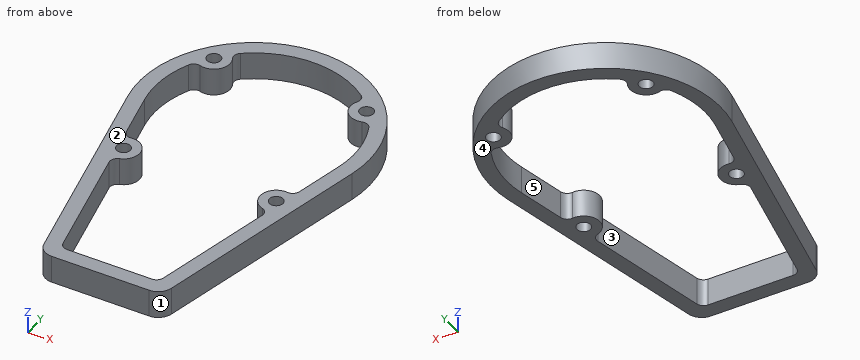
from build123d import *

# Parameters (mm, degrees)
SKETCH3_R           = 4.5
BOSS_EXTRUDE1_DEPTH = 18
FILLET1_R           = 5
FILLET2_R           = 5


with BuildPart() as part:
    # Sketch3 → Boss-Extrude1 (new body)
    with BuildSketch(Plane.XY):
        with BuildLine():
            Line((-31.929873349, -122.5), (31.929873349, -122.5))
            ThreePointArc((31.929873349, -122.5), (38.210043039, -120.281996444), (41.704324989, -114.611893732))
            Line((41.704324989, -114.611893732), (73.308387301, 31.660797012))
            ThreePointArc((73.308387301, 31.660797012), (0, 122.5), (-73.308387301, 31.660797012))
            Line((-73.308387301, 31.660797012), (-41.704324989, -114.611893732))
            ThreePointArc((-41.704324989, -114.611893732), (-38.210043039, -120.281996444), (-31.929873349, -122.5))
        make_face()
        with Locations((50, -12.5)):
            Circle(SKETCH3_R, mode=Mode.SUBTRACT)
        with Locations((50, 87.5)):
            Circle(SKETCH3_R, mode=Mode.SUBTRACT)
        with Locations((-50, 87.5)):
            Circle(SKETCH3_R, mode=Mode.SUBTRACT)
        with Locations((-50, -12.5)):
            Circle(SKETCH3_R, mode=Mode.SUBTRACT)
        with BuildLine():
            Line((-31.929873349, -112.5), (-51.284518999, -22.921132901))
            ThreePointArc((-51.284518999, -22.921132901), (-39.736825778, -10.282511582), (-55.472323677, -3.538768301))
            Line((-55.472323677, -3.538768301), (-63.533935661, 33.772690744))
            ThreePointArc((-63.533935661, 33.772690744), (-64.271528905, 57.204152316), (-56.648842383, 79.373322021))
            ThreePointArc((-56.648842383, 79.373322021), (-41.800877501, 80.940702001), (-43.531035666, 95.770580418))
            ThreePointArc((-43.531035666, 95.770580418), (0, 112.5), (43.531035666, 95.770580418))
            ThreePointArc((43.531035666, 95.770580418), (41.800877501, 80.940702001), (56.648842383, 79.373322021))
            ThreePointArc((56.648842383, 79.373322021), (64.271528905, 57.204152316), (63.533935661, 33.772690744))
            Line((63.533935661, 33.772690744), (55.472323677, -3.538768301))
            ThreePointArc((55.472323677, -3.538768301), (39.736825778, -10.282511582), (51.284518999, -22.921132901))
            Line((51.284518999, -22.921132901), (31.929873349, -112.5))
            Line((31.929873349, -112.5), (-31.929873349, -112.5))
        make_face(mode=Mode.SUBTRACT)
    extrude(amount=BOSS_EXTRUDE1_DEPTH)

    # Fillet1
    fillet1_edges = [part.edges().sort_by_distance(p)[0] for p in [
        (-31.929873349, -112.5, 9),
        (31.929873349, -112.5, 9),
    ]]
    fillet(fillet1_edges, radius=FILLET1_R)

    # Fillet2
    fillet2_edges = [part.edges().sort_by_distance(p)[0] for p in [
        (51.284518999, -22.921132901, 9),
        (55.472323677, -3.538768301, 9),
        (56.648842383, 79.373322021, 9),
        (43.531035666, 95.770580418, 9),
        (-43.531035666, 95.770580418, 9),
        (-56.648842383, 79.373322021, 9),
        (-55.472323677, -3.538768301, 9),
        (-51.284518999, -22.921132901, 9),
    ]]
    fillet(fillet2_edges, radius=FILLET2_R)


solid = part.part
Can you work these out from the model? Positions are in its coordinate system, mm. Face numbers are marked on the shaded views. A direction names the side the tool comes from. Give positions to 0.01 mm unless a question says otherwise; leave off trailing zeros. Loops run counter-clockwise (first coordinate to the right, second up) from the corner with the lowest first, then second, coordinate; pieces in that order, holes last. Notation, with made-up numbers: M 77.25,69.25 L 115.25,69.25 A25 cw 115.25,88.25 Z; hole C 30.5,32 d6. An arc over 180 degrees is marked long. One line per item, written item: value. Start each with the question number.
1) On a 3-axis mill with a long thin cutter (end or side, diameter ignored), from which of +Z, -Z, +X, -X, +Y, -Y can I reach the whole of each face in a straight line? I mean the marked faces 4 and 5. Say none if no direction works.
2) I'm going to push flat-ended pins straight in: pin 1 (4 mm diameter, centred on x = 49, y = 85.5, fed in from -Z); pin 2 (3 mm diameter, centred on y = -88.5, z = 14.5, fed in from -X); pin 3 (2 mm diameter, centred on y = 37, z = 9.5, fed in from +X); pin 4 (6 mm diameter, centred on y = -26.5, z = 13, fed in from -X). Where does each tip first touch, or does it pass through?
3) If we section it at A-A, the plane y = 47.5: Write out the boundary of the cut face in (x, z), and give its area (3 significant figures).
4) If I drill on line 1 (X direction, y = 8.5, z = 8.5); line 2 (Y direction, x = 30.5, z = 17.25); line 3 (X direction, y = -40.5, z = 8.75), over which ranges is the centre line in solid material (lowest first)? Write a range as [from, to].
5) If we section it at B-B, the plane x = 0: Write out the boundary of the cut face in (y, z).
6) If we section it at D-D, the plane z = 6: Give the number of separate pieces and of enclosed holes in the cut face, and give its area (3 significant figures).
7) Thinking about a two-plate mould opening in X: for the marked faces 1, 2 and 3, which applies, +X half, -X half, draft (parallel to the pull), parting line (faces both ways), or undercut?
8) If we section it at C-C, the plane y = 87.5: Write out the boundary of the cut face in (x, z).
Completed:
1. face 4: -Z, +X, -X, +Y, -Y
1. face 5: +Z, -Z
2. pin 1: passes through
2. pin 2: stops at x = -47.67
2. pin 3: stops at x = 74.4
2. pin 4: stops at x = -61.39
3. outline: M -75,0 L -65,0 L -65,18 L -75,18 Z; M 65,0 L 75,0 L 75,18 L 65,18 Z
3. area: 360 mm^2
4. line 1: x = [-68.3, -58.07], [58.07, 68.3]
4. line 2: y = [-122.5, -111.77], [104.9, 116.02]
4. line 3: x = [-57.72, -47.49], [47.49, 57.72]
5. outline: M -122.5,0 L -112.5,0 L -112.5,18 L -122.5,18 Z; M 112.5,0 L 122.5,0 L 122.5,18 L 112.5,18 Z
6. separate pieces: 1
6. enclosed holes: 5
6. area: 6,920 mm^2
7. face 1: +X half
7. face 2: draft
7. face 3: undercut
8. outline: M -63.44,0 L -54.5,0 L -54.5,18 L -63.44,18 Z; M -45.5,0 L -39.5,0 L -39.5,18 L -45.5,18 Z; M 39.5,0 L 45.5,0 L 45.5,18 L 39.5,18 Z; M 54.5,0 L 63.44,0 L 63.44,18 L 54.5,18 Z
